Geometry: final body of the model. Coordinates: model frame, mm. Face numbers are marked on the shaded views. A direction names the side the tool comes from. Round coordinates to 2 decimals unless told otherwise and drop trailing zeros. Loops run counter-clockwise (first coordinate to the right, second up) from the corner with the lowest first, then second, coordinate; pieces in that order, holes last. Notation, with made-up numbers: M 73,59 L 88,59 A27 ccw 88,83 Z; hole C -9,15 d6. An arc over 180 degrees is marked long. Answer as a JSON object with one key per item and string values.
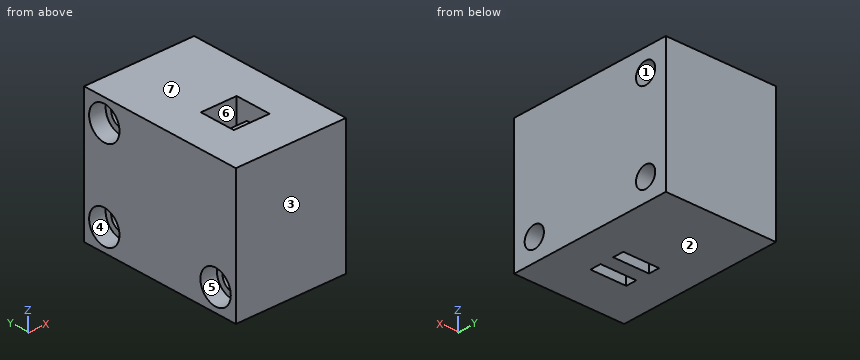
from build123d import *

# Parameters (mm, degrees)
SKETCH020_W     = 20
SKETCH020_H     = 30
PAD007_DEPTH    = 40
SKETCH019_R     = 1.9
POCKET013_DEPTH = 20.001
SKETCH021_R     = 3
POCKET012_DEPTH = 3
SKETCH022_R     = 0.5
POCKET014_DEPTH = 0.5
SKETCH023_W     = 30
SKETCH023_H     = 16
POCKET015_DEPTH = 20.001
SKETCH024_W     = 6.5
SKETCH024_H     = 6.5
POCKET016_DEPTH = 3
SKETCH025_W     = 6.5
SKETCH025_H     = 2
POCKET017_DEPTH = 21.001


with BuildPart() as part:
    # Sketch020 → Pad007 (new body)
    with BuildSketch(Plane.XY):
        with Locations((-43, 0)):
            Rectangle(SKETCH020_W, SKETCH020_H)
    extrude(amount=PAD007_DEPTH)

    # Sketch019 (on Face4 of Pad007) → Pocket013 (cut, through all)
    with BuildSketch(Plane(origin=(-53, 0, 0), x_dir=(0, -1, 0), z_dir=(-1, 0, 0))):
        with Locations((-11, 36)):
            Circle(SKETCH019_R)
        with Locations((11, 20)):
            Circle(SKETCH019_R)
        with Locations((-11, 20)):
            Circle(SKETCH019_R)
        with Locations((-11, 4)):
            Circle(SKETCH019_R)
        with Locations((11, 4)):
            Circle(SKETCH019_R)
    extrude(amount=-POCKET013_DEPTH, mode=Mode.SUBTRACT)

    # Sketch021 (on Face2 of Pocket013) → Pocket012 (cut)
    with BuildSketch(Plane(origin=(-53, 0, 0), x_dir=(0, -1, 0), z_dir=(-1, 0, 0))):
        with Locations((-11, 36)):
            Circle(SKETCH021_R)
        with Locations((-11, 20)):
            Circle(SKETCH021_R)
        with Locations((-11, 4)):
            Circle(SKETCH021_R)
        with Locations((11, 4)):
            Circle(SKETCH021_R)
        with Locations((11, 20)):
            Circle(SKETCH021_R)
    extrude(amount=-POCKET012_DEPTH, mode=Mode.SUBTRACT)

    # Sketch022 (on Face5 of Pocket012) → Pocket014 (cut)
    with BuildSketch(Plane.XY.offset(40)):
        with Locations((-43, -4)):
            Circle(SKETCH022_R)
    extrude(amount=-POCKET014_DEPTH, mode=Mode.SUBTRACT)

    # Sketch023 (on Face2 of Pocket014) → Pocket015 (cut, through all)
    with BuildSketch(Plane(origin=(-53, 0, 0), x_dir=(0, -1, 0), z_dir=(-1, 0, 0))):
        with Locations((0, 8)):
            Rectangle(SKETCH023_W, SKETCH023_H)
    extrude(amount=-POCKET015_DEPTH, mode=Mode.SUBTRACT)

    # Sketch024 (on Face4 of Pocket015) → Pocket016 (cut)
    with BuildSketch(Plane.XY.offset(40)):
        with Locations((-43, -4)):
            Rectangle(SKETCH024_W, SKETCH024_H)
    extrude(amount=-POCKET016_DEPTH, mode=Mode.SUBTRACT)

    # Sketch025 (on Face20 of Pocket016) → Pocket017 (cut, through all)
    with BuildSketch(Plane.XY.offset(37)):
        with Locations((-43, -1.75)):
            Rectangle(SKETCH025_W, SKETCH025_H)
        with Locations((-43, -6.25)):
            Rectangle(SKETCH025_W, SKETCH025_H)
    extrude(amount=-POCKET017_DEPTH, mode=Mode.SUBTRACT)


solid = part.part
1) Pin query (flat end, axial travel): P1, Ø1.2, axis at x = -42, y = -4, coming from the +Z side; P2, Ø7, axis at y = 11, z = 36, coming from the -X side; P3, Ø3.5, axis at y = -11, z = 20, coming from the -X side; P4, Ø1.8, axis at y = -12, z = 21, coming from the -X side. Return the tip coordinate at first contact, or that it passes through.
Results:
{"P1": "z = 37", "P2": "x = -53", "P3": "through", "P4": "x = -50"}
2) Section query B-B (y = -11). Return the cut outline in (x, z).
Results:
{"outline": "M -53,16 L -33,16 L -33,18.1 L -50,18.1 L -50,17 L -53,17 Z; M -53,23 L -50,23 L -50,21.9 L -33,21.9 L -33,40 L -53,40 Z"}
3) Ray query, line 1 (Z direction, x = -41.5, y = 11); line 2 (Z direction, x = -51.5, y = -11); line 3 (Y direction, x = -44.25, z = 23). Return the intervals inside material, ascending.
Results:
{"line 1": "16 to 18.1, 21.9 to 34.1, 37.9 to 40", "line 2": "16 to 17, 23 to 40", "line 3": "-15 to -7.25, -5.25 to -2.75, -0.75 to 15"}
4) Pull-direction query (Y, two-part tool) for the marked faces 1, 2, 3 and 4; classes: +Y half, -Y half, draft (parallel to the pull), parting line (faces both ways), or undercut.
Results:
{"face 1": "undercut", "face 2": "draft", "face 3": "-Y half", "face 4": "undercut"}
5) Section query D-D (z = 36). Return the cut outline in (x, y).
Results:
{"outline": "M -53,-15 L -33,-15 L -33,9.1 L -50,9.1 L -50,8 L -53,8 Z; M -53,14 L -50,14 L -50,12.9 L -33,12.9 L -33,15 L -53,15 Z; hole M -46.25,-7.25 L -39.75,-7.25 L -39.75,-5.25 L -46.25,-5.25 Z; hole M -46.25,-2.75 L -39.75,-2.75 L -39.75,-0.75 L -46.25,-0.75 Z"}
6) Reachability of the marked faces 5, 6 and 7 from +Z, -Z, +X, -X, +Y, -Y: full face, straight path, thin tool, end or side. Return the list, or none.
Results:
{"face 5": "-X", "face 6": "+Z, -Z", "face 7": "+Z, +X, -X, +Y, -Y"}
7) Section query A-A (z = 20). Return the cut outline in (x, y), and give its area (3 significant figures).
Results:
{"outline": "M -53,-15 L -33,-15 L -33,-12.9 L -50,-12.9 L -50,-14 L -53,-14 Z; M -53,-8 L -50,-8 L -50,-9.1 L -33,-9.1 L -33,9.1 L -50,9.1 L -50,8 L -53,8 Z; M -53,14 L -50,14 L -50,12.9 L -33,12.9 L -33,15 L -53,15 Z; hole M -46.25,-7.25 L -39.75,-7.25 L -39.75,-5.25 L -46.25,-5.25 Z; hole M -46.25,-2.75 L -39.75,-2.75 L -39.75,-0.75 L -46.25,-0.75 Z", "area": "409 mm2"}
8) Section query C-C (y = 11). Return the cut outline in (x, z), and give its area (3 significant figures).
Results:
{"outline": "M -53,16 L -33,16 L -33,18.1 L -50,18.1 L -50,17 L -53,17 Z; M -53,23 L -50,23 L -50,21.9 L -33,21.9 L -33,34.1 L -50,34.1 L -50,33 L -53,33 Z; M -53,39 L -50,39 L -50,37.9 L -33,37.9 L -33,40 L -53,40 Z", "area": "315 mm2"}
